```python
from build123d import *

# Parameters (mm, degrees)
REVOLVE_1_ANGLE     = 120
SKETCH_3_R          = 2.5
CUT_EXTRUDE_1_DEPTH = 1.5
FILLET_1_R          = 0.5


with BuildPart() as part:
    # 스케치2 → 회전1 (revolve)
    with BuildSketch(Plane(origin=(0, 0, 0), x_dir=(1, 0, 0), z_dir=(0, 1, 0))):
        Polygon((3.025, -30), (2.025, -30), (2.025, -6), (1.975, -5.95), (1.975, -5.05), (2.025, -5), (2.025, 0), (2.471154323, 0), (3.896197522, -9.284948012), (4.95, -9.76632184), (4.95, -13.919413001), (4.247678793, -13.919413001), (3.896197522, -11.490595407), (3.114172222, -11.490595407), (3.114172222, -18.601840787), (4.95, -19.404070604), (4.95, -21.401570634), (4.273015674, -21.401570634), (4.095786722, -20.253069256), (3.446467915, -20), align=None)
    revolve(axis=Axis((0, 0, 0), (0, 0, 1)), revolution_arc=REVOLVE_1_ANGLE)

    # 스케치3 → 컷-돌출1 (cut)
    with BuildSketch(Plane.XY.offset(30)):
        Circle(SKETCH_3_R)
    extrude(amount=-CUT_EXTRUDE_1_DEPTH, mode=Mode.SUBTRACT)

    # 필렛1
    fillet_1_edges = [part.edges().sort_by_distance(p)[0] for p in [
        (2.475, 4.286825749, 13.919413001),
        (2.475, 4.286825749, 21.401570634),
    ]]
    fillet(fillet_1_edges, radius=FILLET_1_R)


solid = part.part
```
The model under review builds one solid part; all positions refer to its coordinate system, in mm. A direction names the side the tool comes from. Round coordinates to 2 decimals unless told otherwise and drop trailing zeros. Loops run counter-clockwise (first coordinate to the right, second up) from the corner with the lowest first, then second, coordinate; pieces in that order, holes last. Notation, with made-up numbers: M 73.25,8 L 120.25,8 A18 cw 120.25,20 Z; hole C 68,81.25 d5. An arc over 180 degrees is marked long. Put each result on its own line as item: value.
Q1. For pin 1 (0.8 mm diameter, centred on x = 1, y = 1.5, fed in from +Z); pin 2 (1.5 mm diameter, centred on x = -1.5, z = 8.5, fed in from -Y), all flat-tipped, find the tip position at first contact; note any pin that passes through.
Result set:
pin 1: stops at z = 28.5
pin 2: stops at y = 1.75
Q2. To check wall thickness, follow L1, parallel to Z at x = 3.5, y = 3.05; L2, parallel to Z at x = 4.25, y = 0.9; L3, parallel to Z at x = 1, y = 1.9. State the ranges of each line that lie inside material, in increasing order.
Result set:
L1: z = 9.63 to 13.88, 19.27 to 21.36
L2: z = 9.49 to 13.92, 19.14 to 21.4
L3: z = 0 to 28.5
Q3. Consider section A-A, the plane x = 0. Give the boundary of the cut face in (y, z) (3 decimals).
Result set:
outline: M 1.975,5.05 L 2.025,5 L 2.025,0 L 2.471,0 L 3.896,9.285 L 4.95,9.766 L 4.95,13.419 A0.5 ccw 4.45,13.919 L 4.248,13.919 L 3.896,11.491 L 3.114,11.491 L 3.114,18.602 L 4.95,19.404 L 4.95,20.902 A0.5 ccw 4.45,21.402 L 4.273,21.402 L 4.096,20.253 L 3.446,20 L 3.025,30 L 2.5,30 L 2.5,28.5 L 2.025,28.5 L 2.025,6 L 1.975,5.95 Z
Q4. Mouldability with a two-part tool opening along X and no side actions: class faces 1 (the conical face through (1.76, 2.95, 18.74)), 2 (the flat face through (2.8, 0, 14.8)), 3 (the cylindrical face through (1.038, 1.739, 17.092)) as released by +X, released by -X, zero draft, split by the parting line, or undercut.
Result set:
face 1: split by the parting line
face 2: zero draft
face 3: undercut
Q5. Machinability: for faces 4 (the cylindrical face through (2.54, 4.25, 20.16)), 5 (the conical face through (2.134, 3.575, 20.692)), 6 (the flat face through (1.08, 2.42, 30)), 7 (the conical face through (2.09, 3.49, 12.69)), 8 (the flat face through (1, 2, 28.5)), which of the approach directions +Z, -Z, +X, -X, +Y, -Y give a long, thin tool a straight path to every point of the face, cutting with its end or side? Answer none if there is none.
Result set:
face 4: +Z, -Z, +Y
face 5: +Z
face 6: +Z, +X, -X, +Y, -Y
face 7: none
face 8: +Z, -Y
